```python
from build123d import *

# Parameters (mm, degrees)
F1_DEPTH = 3.175


with BuildPart() as f1:
    # F0 (on Top) → F1 (new body)
    with BuildSketch(Plane.XY):
        with BuildLine():
            ThreePointArc((40.786538, 10.257692), (40.208519, 16.222346), (34.925, 19.05))
            Line((34.925, 19.05), (0.141111, 19.05))
            Line((0.141111, 19.05), (-0.141111, 19.05))
            Line((-0.141111, 19.05), (-34.925, 19.05))
            ThreePointArc((-34.925, 19.05), (-40.208519, 16.222346), (-40.786538, 10.257692))
            Line((-40.786538, 10.257692), (-29.698462, -16.353692))
            ThreePointArc((-29.698462, -16.353692), (-29.604894, -16.467341), (-29.464, -16.51))
            Line((-29.464, -16.51), (-25.347444, -16.51))
            ThreePointArc((-25.347444, -16.51), (-25.167839, -16.584395), (-25.093444, -16.764))
            Line((-25.093444, -16.764), (-25.093444, -19.05))
            Line((-25.093444, -19.05), (-0.141111, -19.05))
            Line((-0.141111, -19.05), (0.141111, -19.05))
            Line((0.141111, -19.05), (25.093444, -19.05))
            Line((25.093444, -19.05), (25.093444, -16.764))
            ThreePointArc((25.093444, -16.764), (25.167839, -16.584395), (25.347444, -16.51))
            Line((25.347444, -16.51), (29.464, -16.51))
            ThreePointArc((29.464, -16.51), (29.604894, -16.467341), (29.698462, -16.353692))
            Line((29.698462, -16.353692), (40.786538, 10.257692))
        make_face()
        with BuildLine():
            Line((-21.759422, -10.836581), (-29.125422, -10.836581))
            ThreePointArc((-29.125422, -10.836581), (-29.664238, -10.613396), (-29.887422, -10.074581))
            Line((-29.887422, -10.074581), (-29.887422, -5.248581))
            ThreePointArc((-29.887422, -5.248581), (-29.664238, -4.709765), (-29.125422, -4.486581))
            Line((-29.125422, -4.486581), (-21.759422, -4.486581))
            ThreePointArc((-21.759422, -4.486581), (-21.220607, -4.709765), (-20.997422, -5.248581))
            Line((-20.997422, -5.248581), (-20.997422, -10.074581))
            ThreePointArc((-20.997422, -10.074581), (-21.220607, -10.613396), (-21.759422, -10.836581))
        make_face(mode=Mode.SUBTRACT)
        with BuildLine():
            Line((21.759422, -4.486581), (29.125422, -4.486581))
            ThreePointArc((29.125422, -4.486581), (29.664238, -4.709765), (29.887422, -5.248581))
            Line((29.887422, -5.248581), (29.887422, -10.074581))
            ThreePointArc((29.887422, -10.074581), (29.664238, -10.613396), (29.125422, -10.836581))
            Line((29.125422, -10.836581), (21.759422, -10.836581))
            ThreePointArc((21.759422, -10.836581), (21.220607, -10.613396), (20.997422, -10.074581))
            Line((20.997422, -10.074581), (20.997422, -5.248581))
            ThreePointArc((20.997422, -5.248581), (21.220607, -4.709765), (21.759422, -4.486581))
        make_face(mode=Mode.SUBTRACT)
        with BuildLine():
            Line((-21.759422, 3.133419), (-35.475422, 3.133419))
            ThreePointArc((-35.475422, 3.133419), (-36.014238, 3.356604), (-36.237422, 3.895419))
            Line((-36.237422, 3.895419), (-36.237422, 13.801419))
            ThreePointArc((-36.237422, 13.801419), (-36.014238, 14.340235), (-35.475422, 14.563419))
            Line((-35.475422, 14.563419), (-21.759422, 14.563419))
            ThreePointArc((-21.759422, 14.563419), (-21.220607, 14.340235), (-20.997422, 13.801419))
            Line((-20.997422, 13.801419), (-20.997422, 3.895419))
            ThreePointArc((-20.997422, 3.895419), (-21.220607, 3.356604), (-21.759422, 3.133419))
        make_face(mode=Mode.SUBTRACT)
        with BuildLine():
            Line((-18.415, -13.9192), (-18.415, 13.9192))
            ThreePointArc((-18.415, 13.9192), (-18.229013, 14.368213), (-17.78, 14.5542))
            Line((-17.78, 14.5542), (-16.51, 14.5542))
            ThreePointArc((-16.51, 14.5542), (-16.060987, 14.368213), (-15.875, 13.9192))
            Line((-15.875, 13.9192), (-15.875, -13.9192))
            ThreePointArc((-15.875, -13.9192), (-16.060987, -14.368213), (-16.51, -14.5542))
            Line((-16.51, -14.5542), (-17.78, -14.5542))
            ThreePointArc((-17.78, -14.5542), (-18.229013, -14.368213), (-18.415, -13.9192))
        make_face(mode=Mode.SUBTRACT)
        with BuildLine():
            Line((-12.7, -13.9192), (-12.7, 13.9192))
            ThreePointArc((-12.7, 13.9192), (-12.514013, 14.368213), (-12.065, 14.5542))
            Line((-12.065, 14.5542), (-10.795, 14.5542))
            ThreePointArc((-10.795, 14.5542), (-10.345987, 14.368213), (-10.16, 13.9192))
            Line((-10.16, 13.9192), (-10.16, -13.9192))
            ThreePointArc((-10.16, -13.9192), (-10.345987, -14.368213), (-10.795, -14.5542))
            Line((-10.795, -14.5542), (-12.065, -14.5542))
            ThreePointArc((-12.065, -14.5542), (-12.514013, -14.368213), (-12.7, -13.9192))
        make_face(mode=Mode.SUBTRACT)
        with BuildLine():
            Line((-6.985, -13.9192), (-6.985, 13.9192))
            ThreePointArc((-6.985, 13.9192), (-6.799013, 14.368213), (-6.35, 14.5542))
            Line((-6.35, 14.5542), (-5.08, 14.5542))
            ThreePointArc((-5.08, 14.5542), (-4.630987, 14.368213), (-4.445, 13.9192))
            Line((-4.445, 13.9192), (-4.445, -13.9192))
            ThreePointArc((-4.445, -13.9192), (-4.630987, -14.368213), (-5.08, -14.5542))
            Line((-5.08, -14.5542), (-6.35, -14.5542))
            ThreePointArc((-6.35, -14.5542), (-6.799013, -14.368213), (-6.985, -13.9192))
        make_face(mode=Mode.SUBTRACT)
        with BuildLine():
            Line((-0.635, 14.5542), (0.635, 14.5542))
            ThreePointArc((0.635, 14.5542), (1.084013, 14.368213), (1.27, 13.9192))
            Line((1.27, 13.9192), (1.27, -13.9192))
            ThreePointArc((1.27, -13.9192), (1.084013, -14.368213), (0.635, -14.5542))
            Line((0.635, -14.5542), (-0.635, -14.5542))
            ThreePointArc((-0.635, -14.5542), (-1.084013, -14.368213), (-1.27, -13.9192))
            Line((-1.27, -13.9192), (-1.27, 13.9192))
            ThreePointArc((-1.27, 13.9192), (-1.084013, 14.368213), (-0.635, 14.5542))
        make_face(mode=Mode.SUBTRACT)
        with BuildLine():
            ThreePointArc((6.35, 14.5542), (6.799013, 14.368213), (6.985, 13.9192))
            Line((6.985, 13.9192), (6.985, -13.9192))
            ThreePointArc((6.985, -13.9192), (6.799013, -14.368213), (6.35, -14.5542))
            Line((6.35, -14.5542), (5.08, -14.5542))
            ThreePointArc((5.08, -14.5542), (4.630987, -14.368213), (4.445, -13.9192))
            Line((4.445, -13.9192), (4.445, 13.9192))
            ThreePointArc((4.445, 13.9192), (4.630987, 14.368213), (5.08, 14.5542))
            Line((5.08, 14.5542), (6.35, 14.5542))
        make_face(mode=Mode.SUBTRACT)
        with BuildLine():
            ThreePointArc((12.065, 14.5542), (12.514013, 14.368213), (12.7, 13.9192))
            Line((12.7, 13.9192), (12.7, -13.9192))
            ThreePointArc((12.7, -13.9192), (12.514013, -14.368213), (12.065, -14.5542))
            Line((12.065, -14.5542), (10.795, -14.5542))
            ThreePointArc((10.795, -14.5542), (10.345987, -14.368213), (10.16, -13.9192))
            Line((10.16, -13.9192), (10.16, 13.9192))
            ThreePointArc((10.16, 13.9192), (10.345987, 14.368213), (10.795, 14.5542))
            Line((10.795, 14.5542), (12.065, 14.5542))
        make_face(mode=Mode.SUBTRACT)
        with BuildLine():
            ThreePointArc((17.78, 14.5542), (18.229013, 14.368213), (18.415, 13.9192))
            Line((18.415, 13.9192), (18.415, -13.9192))
            ThreePointArc((18.415, -13.9192), (18.229013, -14.368213), (17.78, -14.5542))
            Line((17.78, -14.5542), (16.51, -14.5542))
            ThreePointArc((16.51, -14.5542), (16.060987, -14.368213), (15.875, -13.9192))
            Line((15.875, -13.9192), (15.875, 13.9192))
            ThreePointArc((15.875, 13.9192), (16.060987, 14.368213), (16.51, 14.5542))
            Line((16.51, 14.5542), (17.78, 14.5542))
        make_face(mode=Mode.SUBTRACT)
        with BuildLine():
            Line((21.759422, 14.563419), (35.475422, 14.563419))
            ThreePointArc((35.475422, 14.563419), (36.014238, 14.340235), (36.237422, 13.801419))
            Line((36.237422, 13.801419), (36.237422, 3.895419))
            ThreePointArc((36.237422, 3.895419), (36.014238, 3.356604), (35.475422, 3.133419))
            Line((35.475422, 3.133419), (21.759422, 3.133419))
            ThreePointArc((21.759422, 3.133419), (21.220607, 3.356604), (20.997422, 3.895419))
            Line((20.997422, 3.895419), (20.997422, 13.801419))
            ThreePointArc((20.997422, 13.801419), (21.220607, 14.340235), (21.759422, 14.563419))
        make_face(mode=Mode.SUBTRACT)
    extrude(amount=F1_DEPTH)


solid = f1.part
```
The model under review builds one solid part; all positions refer to its coordinate system, in mm. A direction names the side the tool comes from. Round coordinates to 2 decimals unless told otherwise and drop trailing zeros.
(1) Wall thickness on L1, parallel to Y at x = 22.5, z = 1.5; L2, parallel to Y at x = 5.5, z = 0.3; L3, parallel to Y at x = 35, z = 1.4: over which ranges is each line inside the solid? List them lowest first.
Working result:
L1: y = -19.05 to -10.84, -4.49 to 3.13, 14.56 to 19.05
L2: y = -19.05 to -14.55, 14.55 to 19.05
L3: y = -3.63 to 3.13, 14.56 to 19.05
(2) Tool access review of faces 4 (the face through (-10, 0, 0)), 5 (the face through (-18.415, 0, 2)): name each direction out of +Z, -Z, +X, -X, +Y, -Y from which nothing blocks a thin tool from reaching the whole face with its end or side.
Working result:
face 4: -Z, +X, -X, +Y, -Y
face 5: +Z, -Z
(3) Mouldability with a two-part tool opening along Y and no side actions: class faces 1 (the face through (-27, -16.51, 2)), 2 (the face through (20.997, 9, 2)), 3 (the face through (-10, 0, 3.175)) as released by +Y, released by -Y, zero draft, split by the parting line, or undercut.
Working result:
face 1: released by -Y
face 2: undercut
face 3: zero draft
(4) Take a section at A-A, the plane y = -2. Count the separate pieces of the cut face and the enclosed holes in it, plus the area to 3 significant figures.
Working result:
separate pieces: 8
enclosed holes: 0
area: 170 mm2
(5) For P1, Ø1, axis at y = -3.5, z = 1.5, coming from the -X side; P2, Ø1, axis at y = -6.5, z = 1.5, coming from the -X side; P3, Ø1.6, axis at y = 7, z = 2, coming from the +X side, all flat-tipped, find the tip position at first contact; note any pin that passes through.
Working result:
P1: stops at x = -35.26
P2: stops at x = -34.01
P3: stops at x = 39.76
